from build123d import *

# Parameters (mm, degrees)
F0_W     = 100
F0_H     = 200
F1_DEPTH = 200
F0_W_2   = 150
F2_DEPTH = 200
F3_W     = 90
F3_H     = 190
F4_DEPTH = 195
F5_W     = 100
F5_H     = 130
F7_DEPTH = 195
F6_W     = 130
F6_H     = 160
F6_W_2   = 100
F6_H_2   = 130
F8_DEPTH = 195


with BuildPart() as f1:
    # F0 (on Top) → F1 (new body)
    with BuildSketch(Plane.XY):
        Rectangle(F0_W, F0_H)
    extrude(amount=F1_DEPTH)

    # F0 (on Top) → F2 (join)
    with BuildSketch(Plane.XY):
        with Locations((125, 0)):
            Rectangle(F0_W_2, F0_H)
    extrude(amount=F2_DEPTH)

    # F3 (on face) → F4 (cut)
    with BuildSketch(Plane.XY.offset(200)):
        Rectangle(F3_W, F3_H)
    extrude(amount=-F4_DEPTH, mode=Mode.SUBTRACT)

    # F5 (on face) → F7 (cut)
    with BuildSketch(Plane.XY.offset(200)):
        with Locations((125, -0.22641)):
            Rectangle(F5_W, F5_H)
    extrude(amount=-F7_DEPTH, mode=Mode.SUBTRACT)

    # F6 (on face) → F8 (cut)
    with BuildSketch(Plane.XY.offset(200)):
        with Locations((125, -0.22641)):
            Rectangle(F6_W, F6_H)
        with Locations((125, -0.22641)):
            Rectangle(F6_W, F6_H)
        with Locations((125, -0.22641)):
            Rectangle(F6_W_2, F6_H_2, mode=Mode.SUBTRACT)
    extrude(amount=-F8_DEPTH, mode=Mode.SUBTRACT)


solid = f1.part
Verification items for the finished model (mm, model axes). A direction names the side the tool comes from. Give positions to 0.01 mm unless a question says otherwise; leave off trailing zeros. Loops run counter-clockwise (first coordinate to the right, second up) from the corner with the lowest first, then second, coordinate; pieces in that order, holes last. Notation, with made-up numbers: (34.25, 77.25) - (74.25, 77.25) arc R15 ccw to (74.25, 98.25) - close; hole circle Ø11 at (12, 89.5). An arc over 180 degrees is marked (long way). Write item = value, one per line. Start each with the question number.
Q1. Thickness scan on line 1 (X direction, y = -67, z = 141); line 2 (Y direction, x = 104, z = 109); line 3 (X direction, y = 88, z = 26). Record the ranges inside material, lowest first.
Q2. Cross-section at D-D, the plane x = 3.5. Enter the section's corners in (y, z).
Q3. Cross-section at A-A, the plane x = 75.5. Enter the section's corners in (y, z).
Q4. Cross-section at B-B, the plane z = 38.5. Enter the section's corners in (x, y), and give its area (3 significant figures).
Q5. Depth check by flat-ended pin: P1, Ø6, axis at x = 9.5, y = 6.5, coming from the +Z side. Enter the tip coordinate at first touch or a pass-through.
Q6. Mould release check, pull along Y, two halves, no side actions. Record for faces 1 (the face through (73, 100, 99)), 2 (the face through (73, -100, 99)), 3 (the face through (124, 79.774, 104)), 4 (the face through (73, 1, 0)): released by +Y, released by -Y, zero draft, split by the parting line, or undercut.
Q7. Tool access check on faces 5 (the face through (-1, -95, 104)), 6 (the face through (200, -1, 99)). Record the directions out of +Z, -Z, +X, -X, +Y, -Y that give a thin tool (end or side, any length) a straight path to the whole face; none if there is none.
Q8. Cross-section at C-C, the plane y = 71.5. Enter the section's corners in (x, z).
Answer key:
q1.line_1 = -50 to -45, 45 to 60, 190 to 200
q1.line_2 = -100 to -80.23, 79.77 to 100
q1.line_3 = -50 to -45, 45 to 200
q2.outline = (-100, 0) - (100, 0) - (100, 200) - (95, 200) - (95, 5) - (-95, 5) - (-95, 200) - (-100, 200) - close
q3.outline = (-100, 0) - (100, 0) - (100, 200) - (79.77, 200) - (79.77, 5) - (-80.23, 5) - (-80.23, 200) - (-100, 200) - close
q4.outline = (-50, -100) - (200, -100) - (200, 100) - (-50, 100) - close; hole (-45, -95) - (45, -95) - (45, 95) - (-45, 95) - close; hole (60, -80.23) - (190, -80.23) - (190, 79.77) - (60, 79.77) - close
q4.area = 12,100 mm^2
q5.P1 = 5
q6.face_1 = released by +Y
q6.face_2 = released by -Y
q6.face_3 = undercut
q6.face_4 = zero draft
q7.face_5 = +Z
q7.face_6 = +Z, -Z, +X, +Y, -Y
q8.outline = (-50, 0) - (200, 0) - (200, 200) - (190, 200) - (190, 5) - (60, 5) - (60, 200) - (45, 200) - (45, 5) - (-45, 5) - (-45, 200) - (-50, 200) - close
